Geometry: see drawing. Coordinates: mm, zero at the bounding-box minimum. A direction names the side the tool comes from. Give positions to 0.01 mm unless a question says otherwise; leave off trailing zeros. Order: outer loops, then holes, each group sorted by start corner. A loop starts at its lowest first (then second) coordinate and runs counter-clockwise, first axis right, second up. Notation, with made-up numbers: M 40,37.25 L 93,37.25 A27 cw 93,64.25 Z; hole C 53.25,9 d7. An arc over 180 degrees is marked long. Use a Markdown table: item, result.
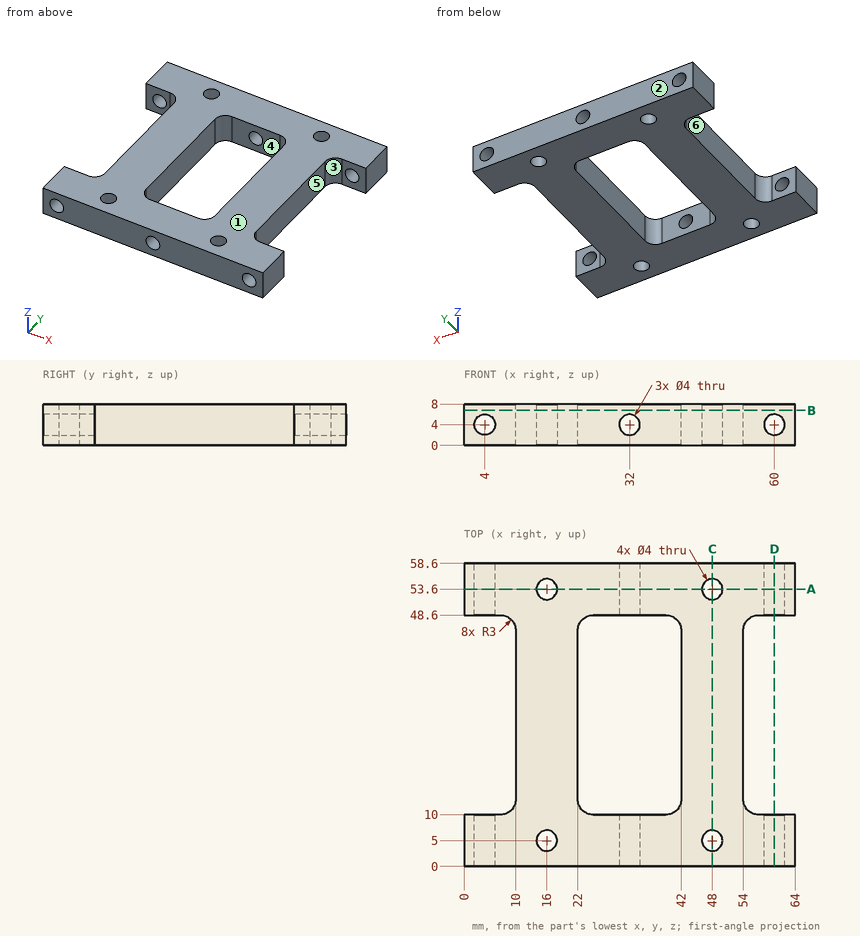
1) Material intervals for line 1 (Y direction, x = 16, z = 4); line 2 (X direction, y = 28, z = 5.5); line 3 (Y direction, x = 3.5, z = 7.25), sorted ascending. Write a range as from..to.
Response values:
| item | result |
|---|---|
| line 1 | y = 0..3, 7..51.6, 55.6..58.6 |
| line 2 | x = 10..22, 42..54 |
| line 3 | y = 0..10, 48.6..58.6 |
2) Cut plane D-D on x = 60. Return loops of the section in (y, z), and give its area (3 significant figures).
Response values:
| item | result |
|---|---|
| outline | M 0,0 L 10,0 L 10,2 L 0,2 Z; M 0,6 L 10,6 L 10,8 L 0,8 Z; M 48.6,0 L 58.6,0 L 58.6,2 L 48.6,2 Z; M 48.6,6 L 58.6,6 L 58.6,8 L 48.6,8 Z |
| area | 80.0 mm² |
3) Reachability of the marked faces 4, 5 and 6 from +Z, -Z, +X, -X, +Y, -Y: full face, straight path, thin tool, end or side. Return the list, or none.
Response values:
| item | result |
|---|---|
| face 4 | +Z, -Z |
| face 5 | +Z, -Z, +X |
| face 6 | +Z, -Z, -X |
4) First-contact query: pin 1 Ø2 at (y, z) = (32, 3.5) entering from +X; pin 2 Ø3 at (x, z) = (4, 4) entering from -Y; pin 3 Ø1.5 at (y, z) = (40.5, 6.5) entering from -X. Flat tips, straight axial feed; report the tip coordinate or a pass-through.
Response values:
| item | result |
|---|---|
| pin 1 | stops at x = 54 |
| pin 2 | passes through |
| pin 3 | stops at x = 10 |
5) Cut plane A-A on y = 53.6. Return loops of the section in (x, z), and give its area (3 significant figures).
Response values:
| item | result |
|---|---|
| outline | M 0,0 L 14,0 L 14,8 L 0,8 Z; M 18,0 L 46,0 L 46,8 L 18,8 Z; M 50,0 L 64,0 L 64,8 L 50,8 Z; hole C 4,4 d4; hole C 32,4 d4; hole C 60,4 d4 |
| area | 410 mm² |
6) Mould query, pull axis Y, two halves, no side actions, for the marked faces 1, 2 and 3. Classes: released by +Y, released by -Y, zero draft, split by the parting line, or undercut.
Response values:
| item | result |
|---|---|
| face 1 | zero draft |
| face 2 | released by +Y |
| face 3 | undercut |
7) Cut plane B-B on z = 6.75. Return loops of the section in (x, y).
Response values:
| item | result |
|---|---|
| outline | M 0,0 L 64,0 L 64,10 L 57,10 A3 cw 54,13 L 54,45.6 A3 cw 57,48.6 L 64,48.6 L 64,58.6 L 0,58.6 L 0,48.6 L 7,48.6 A3 cw 10,45.6 L 10,13 A3 cw 7,10 L 0,10 Z; hole C 16,5 d4; hole C 16,53.6 d4; hole M 22,13 A3 ccw 25,10 L 39,10 A3 ccw 42,13 L 42,45.6 A3 ccw 39,48.6 L 25,48.6 A3 ccw 22,45.6 Z; hole C 48,5 d4; hole C 48,53.6 d4 |
8) Cut plane C-C on x = 48. Return loops of the section in (y, z), and give its area (3 significant figures).
Response values:
| item | result |
|---|---|
| outline | M 0,0 L 3,0 L 3,8 L 0,8 Z; M 7,0 L 51.6,0 L 51.6,8 L 7,8 Z; M 55.6,0 L 58.6,0 L 58.6,8 L 55.6,8 Z |
| area | 405 mm² |
